Build history of the part. All positions in model axes, mm. A direction names the side the tool comes from. Round coordinates to 2 decimals unless told otherwise and drop trailing zeros. Order: outer loops, then holes, each group sorted by start corner. A loop starts at its lowest first (then second) coordinate and runs counter-clockwise, first axis right, second up. Notation, with made-up numbers: (32, 50) -> (36, 50) arc R25 ccw to (36, 68) -> close; hole circle Ø8 at (-20, -27). An arc over 180 degrees is marked (long way). Use a Markdown table: item, result. Add a question column.
Item 1: Two-plate mould, pull along X, no slides. Class faces 3 (the face through (39, 2, 0)), 4 (the face through (73.986, 2.413, -84.297)), 5 (the face through (25, 2.4, -49.1)): released by +X, released by -X, zero draft, split by the parting line, or undercut.
Item 2: Slice it at B-B, the plane x = 25. Give the cut face in (y, z), plus the area to 3 significant figures.
Item 3: Probe L1, parallel to X at y = 3.45, z = -12.5; L2, parallel to X at y = 1.4, z = -53.5; L3, parallel to Z at x = 25, y = 2.8. List the from-to ranges inside material, lowest first.
Item 4: 3-axis set-ups, long thin cutter, end or side, ignore diameter. For faces 1 (the face through (5.703, 2.413, -83.986)), 2 (the face through (23.6, 2, -53)): which of +Z, -Z, +X, -X, +Y, -Y reach the whole face in a straight line?
Item 5: Slice it at A-A, the plane z = -12.5. Give the cut face in (x, y).
Item 6: Slice it at D-D, the plane x = 10. Give the cut face in (y, z).
Item 7: Pin check, flat tip, straight feed: pin 1 (12 mm diameter, centred on x = 67.5, z = -56.5, fed in from -Y). Stop position of the tip, or through.
Item 8: Slice it at C-C, the plane y = 3.15. Give the cut face in (x, z).
from build123d import *

# Parameters (mm, degrees)
SKETCH1_W           = 80
SKETCH1_H           = 90
BOSS_EXTRUDE1_DEPTH = 4.76
SKETCH2_R           = 1.65
SKETCH2_R_2         = 1.4
CUT_EXTRUDE1_DEPTH  = 5.76
FILLET1_R           = 20


with BuildPart() as part:
    # Sketch1 → Boss-Extrude1 (new body)
    with BuildSketch(Plane(origin=(0, 0, 0), x_dir=(1, 0, 0), z_dir=(0, 1, 0))):
        with Locations((40, 45)):
            Rectangle(SKETCH1_W, SKETCH1_H)
    extrude(amount=BOSS_EXTRUDE1_DEPTH)

    # Sketch2 → Cut-Extrude1 (cut, through all)
    with BuildSketch(Plane(origin=(0, 4.76, 0), x_dir=(1, 0, 0), z_dir=(0, 1, 0))):
        with Locations((10, 12.5)):
            Circle(SKETCH2_R)
        with Locations((70, 12.5)):
            Circle(SKETCH2_R)
        with Locations((25, 83)):
            Circle(SKETCH2_R_2)
        with Locations((55, 83)):
            Circle(SKETCH2_R_2)
        with BuildLine():
            Line((26.4, 55.5), (26.4, 50.5))
            ThreePointArc((26.4, 50.5), (25, 49.1), (23.6, 50.5))
            Line((23.6, 50.5), (23.6, 55.5))
            ThreePointArc((23.6, 55.5), (25, 56.9), (26.4, 55.5))
        make_face()
        with BuildLine():
            Line((53.6, 55.5), (53.6, 50.5))
            ThreePointArc((53.6, 50.5), (55, 49.1), (56.4, 50.5))
            Line((56.4, 50.5), (56.4, 55.5))
            ThreePointArc((56.4, 55.5), (55, 56.9), (53.6, 55.5))
        make_face()
    extrude(amount=-CUT_EXTRUDE1_DEPTH, mode=Mode.SUBTRACT)

    # Fillet1
    fillet1_edges = [part.edges().sort_by_distance(p)[0] for p in [
        (0, 2.38, -90),
        (80, 2.38, -90),
    ]]
    fillet(fillet1_edges, radius=FILLET1_R)


solid = part.part
Check sheet entries:
| question | item | result |
|---|---|---|
| 1 | face 3 | zero draft |
| 1 | face 4 | released by +X |
| 1 | face 5 | undercut |
| 2 | outline | (0, -90) -> (4.76, -90) -> (4.76, -84.4) -> (0, -84.4) -> close; (0, -81.6) -> (4.76, -81.6) -> (4.76, -56.9) -> (0, -56.9) -> close; (0, -49.1) -> (4.76, -49.1) -> (4.76, 0) -> (0, 0) -> close |
| 2 | area | 378 mm2 |
| 3 | L1 | 0 to 8.35, 11.65 to 68.35, 71.65 to 80 |
| 3 | L2 | 0 to 23.6, 26.4 to 53.6, 56.4 to 80 |
| 3 | L3 | -90 to -84.4, -81.6 to -56.9, -49.1 to 0 |
| 4 | face 1 | -Z, -X, +Y, -Y |
| 4 | face 2 | +Y, -Y |
| 5 | outline | (0, 0) -> (8.35, 0) -> (8.35, 4.76) -> (0, 4.76) -> close; (11.65, 0) -> (68.35, 0) -> (68.35, 4.76) -> (11.65, 4.76) -> close; (71.65, 0) -> (80, 0) -> (80, 4.76) -> (71.65, 4.76) -> close |
| 6 | outline | (0, -87.32) -> (4.76, -87.32) -> (4.76, -14.15) -> (0, -14.15) -> close; (0, -10.85) -> (4.76, -10.85) -> (4.76, 0) -> (0, 0) -> close |
| 7 | pin 1 | y = 0 |
| 8 | outline | (0, -70) arc R20 ccw to (20, -90) -> (60, -90) arc R20 ccw to (80, -70) -> (80, 0) -> (0, 0) -> close; hole circle Ø3.3 at (10, -12.5); hole circle Ø2.8 at (25, -83); hole (23.6, -55.5) arc R1.4 ccw to (26.4, -55.5) -> (26.4, -50.5) arc R1.4 ccw to (23.6, -50.5) -> close; hole circle Ø2.8 at (55, -83); hole (53.6, -55.5) arc R1.4 ccw to (56.4, -55.5) -> (56.4, -50.5) arc R1.4 ccw to (53.6, -50.5) -> close; hole circle Ø3.3 at (70, -12.5) |
